Input: part model. Units: mm. Frame: model coordinates. Face numbers are marked on the shaded views. A direction names the side the tool comes from. Give positions to 0.01 mm unless a question says otherwise; leave off trailing zeros. Order: outer loops, then holes, each group sorted by start corner. A loop starts at its lowest first (then second) coordinate and runs counter-clockwise, first axis right, second up. Notation, with made-up numbers: (59.25, 51) - (82.25, 51) arc R25 cw to (82.25, 90) - close; hole circle Ø4 at (-11.5, 14.5). An arc over 180 degrees is marked (long way). Use a Markdown table: item, result.
Autodesk Inventor part; units mm, degrees
ref_plane "YZ Plane" through (0, 0, 0) normal (1, 0, 0) x (0, 1, 0)
ref_plane "XZ Plane" through (0, 0, 0) normal (0, 1, 0) x (-1, 0, 0)
ref_plane "XY Plane" through (0, 0, 0) normal (0, 0, 1) x (1, 0, 0)
sketch "Sketch1" plane through (0, 0, 0) normal (0, 0, 1) x (1, 0, 0)
  circle A0 centre (0, 0) radius 15
  circle A1 centre (0, 0) radius 20
  circle A2 centre (0, 0) radius 32.5
  circle A3 centre (0, 0) radius 50
  dimension "d0" = 30
  dimension "d1" = 40
  dimension "d2" = 65
  dimension "d3" = 100
extrude "Extrusion1" add sketch "Sketch1" along normal blind 10 contours A2 | A3
extrude "Extrusion2" add sketch "Sketch1" along normal blind 20 contours A1
extrude "Extrusion3" add sketch "Sketch1" along normal blind 15 contours A2
fillet "Fillet1" radius 5 1 edges at (-20, 0, 15)
extrude "Extrusion4" add sketch "Sketch1" against normal blind 2 contours A1 | A2
sketch "Sketch2" plane through (0, 0, 10) normal (0, 0, 1) x (1, 0, 0)
  point P0 (0, 0)
  point P1 (0, 41)
  point P2 (28.9914, 28.9914)
  point P3 (41, 0)
  point P4 (28.9914, -28.9914)
  point P5 (0, -41)
  point P6 (-28.9914, -28.9914)
  point P7 (-41, 0)
  point P8 (-28.9914, 28.9914)
  dimension "d13" = 41
  dimension "d16" = 360
hole "Hole1" at (0, 41, 10) at (28.9914, 28.9914, 10) at (41, 0, 10) at (28.9914, -28.9914, 10) at (0, -41, 10) at (-28.9914, -28.9914, 10) at (-41, 0, 10) at (-28.9914, 28.9914, 10) direction (0, 0, -1) diameter 8.5 depth 26 tip angle 118
properties part number "Part11_CPY"
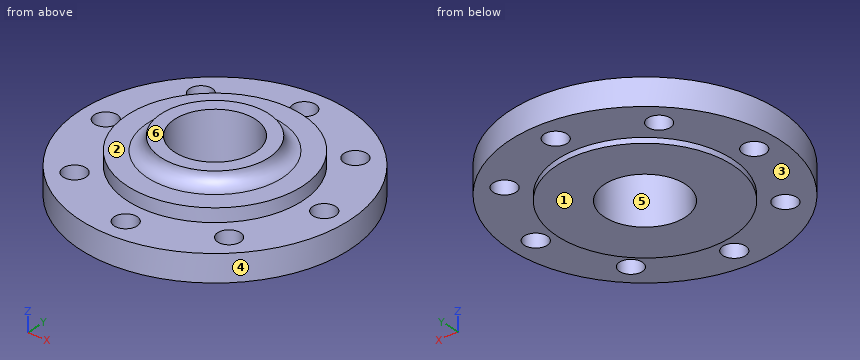
1. Section query C-C (y = -39). Return loops of the section in (x, z), then the cut area to 3 significant figures.
Response:
| item | result |
|---|---|
| outline | (-31.29, 0) - (-3.75, 0) - (-3.75, 10) - (-31.29, 10) - close; (3.75, 0) - (31.29, 0) - (31.29, 10) - (3.75, 10) - close |
| area | 551 mm^2 |
2. Material intervals for line 1 along Y through (x, z) = (0, 5.75); line 2 along Y through (x, z) = (1, 9.5); line 3 along X through (y, z) = (-31, 4), sorted ascending.
Response:
| item | result |
|---|---|
| line 1 | y = -50 to -45.25, -36.75 to -15, 15 to 36.75, 45.25 to 50 |
| line 2 | y = -49.99 to -45.13, -36.87 to -14.97, 14.97 to 36.87, 45.13 to 49.99 |
| line 3 | x = -39.23 to -32.74, -25.25 to 25.25, 32.74 to 39.23 |
3. Pin query (flat end, axial travel): pin 1 (1 mm diameter, centred on y = -14.5, z = 6, fed in from -X); pin 2 (11 mm diameter, centred on x = 41, y = 0, fed in from +Z); pin 3 (13.5 mm diameter, centred on x = -28.99, y = 28.99, fed in from -Z). Return the tip coordinate at first contact, or that it passes through.
Response:
| item | result |
|---|---|
| pin 1 | stops at x = -48 |
| pin 2 | stops at z = 10 |
| pin 3 | stops at z = 0 |
4. Set-up query: the marked faces 1, 2 and 3. Return all of +Z, -Z, +X, -X, +Y, -Y with unobstructed straight access to the full face (end or side cutting, diameter ignored); none if empty.
Response:
| item | result |
|---|---|
| face 1 | -Z, +X, -X, +Y, -Y |
| face 2 | +Z |
| face 3 | -Z |
5. Section query A-A (y = 0). State how many separate pieces and enclosed holes the cut face has, then the cut area to 3 significant figures.
Response:
| item | result |
|---|---|
| separate pieces | 4 |
| enclosed holes | 0 |
| area | 836 mm^2 |
6. Mould query, pull axis X, two halves, no side actions, for the marked faces 4, 5 and 6. Classes: pulls with the +X half, pulls with the -X half, needs draft (parallel to the pull), parting line crosses it, or undercut.
Response:
| item | result |
|---|---|
| face 4 | parting line crosses it |
| face 5 | undercut |
| face 6 | needs draft |
7. Section query B-B (x = -41). Return loops of the section in (y, z), then the cut area to 3 significant figures.
Response:
| item | result |
|---|---|
| outline | (-28.62, 0) - (-4.25, 0) - (-4.25, 10) - (-28.62, 10) - close; (4.25, 0) - (28.62, 0) - (28.62, 10) - (4.25, 10) - close |
| area | 487 mm^2 |
